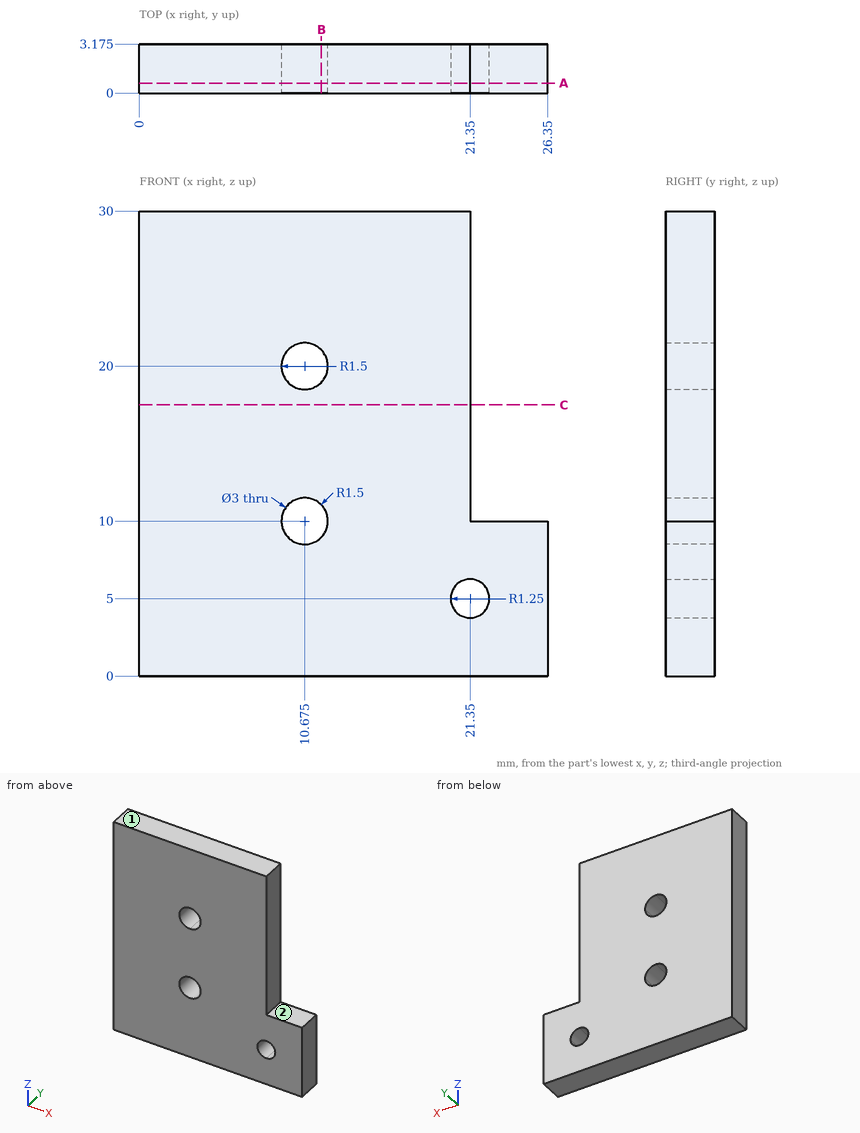
The figure shows three views and two pictorial views of one solid part (mm, origin at its lowest corner). Answer the questions. A direction names the side the tool comes from. Give positions to 0.01 mm unless a question says otherwise; leave off trailing zeros. Order: outer loops, then holes, each group sorted by start corner. A loop starts at its lowest first (then second) coordinate and runs counter-clockwise, first axis right, second up. Notation, with made-up numbers: (-1.5, 14.25) -> (15.5, 14.25) arc R11 ccw to (15.5, 33.25) -> close; hole circle Ø7 at (22.25, -12). An arc over 180 degrees is marked (long way). Answer as a JSON object with one key per item and string values. Group by question number.
Item 1: The part is cut by section B-B on x = 11.75. Write down the section's boundary in (y, z) (3 decimals).
Item 2: The part is cut by section A-A on y = 0.65. Write down the section's boundary in (x, z) (3 decimals).
Item 3: A tool of negligible diameter and unlimited length cuts with its end or side. For the marked faces 1 and 2, from which of +Z, -Z, +X, -X, +Y, -Y can it reach the whole face along a straight path? Write none if from no direction.
Item 4: Flat-ended cylindrical pins translate along their axes: pin 1 (1.6 mm diameter, centred on y = 2, z = 20.5, fed in from +X); pin 2 (2.5 mm diameter, centred on x = 10.675, z = 10, fed in from +Y); pin 3 (1 mm diameter, centred on x = 25, y = 1, fed in from +Z). Find the tip coordinate at first contact, or state that the pin passes through.
Item 5: Consider L1, parallel to Z at x = 12, y = 3; L2, parallel to X at y = 2.1, z = 5; L3, parallel to X at y = 0.2, z = 14.5. Determine where each line is inside the solid, lowest interval first. Write a range as from..to.
Item 6: The part is cut by section C-C on z = 17.5. Write down the section's boundary in (x, y) (3 decimals).
Result set:
{
 "1": {"outline": "(0, 0) -> (3.175, 0) -> (3.175, 8.954) -> (0, 8.954) -> close; (0, 11.046) -> (3.175, 11.046) -> (3.175, 18.954) -> (0, 18.954) -> close; (0, 21.046) -> (3.175, 21.046) -> (3.175, 30) -> (0, 30) -> close"},
 "2": {"outline": "(0, 0) -> (26.35, 0) -> (26.35, 10) -> (21.35, 10) -> (21.35, 30) -> (0, 30) -> close; hole circle Ø3 at (10.675, 10); hole circle Ø3 at (10.675, 20); hole circle Ø2.5 at (21.35, 5)"},
 "3": {"face 1": "+Z, +X, -X, +Y, -Y", "face 2": "+Z, +X, +Y, -Y"},
 "4": {"pin 1": "x = 21.35", "pin 2": "through", "pin 3": "z = 10"},
 "5": {"L1": "0..9.3, 10.7..19.3, 20.7..30", "L2": "0..20.1, 22.6..26.35", "L3": "0..21.35"},
 "6": {"outline": "(0, 0) -> (21.35, 0) -> (21.35, 3.175) -> (0, 3.175) -> close"}
}
